Verification items for the finished model (mm, model axes). Face numbers are marked on the shaded views. A direction names the side the tool comes from. Round coordinates to 2 decimals unless told otherwise and drop trailing zeros. Write each loop counter-clockwise with the first axis right and the second up, starting at its lowest first coordinate (ties: lowest second). Pieces come first, ordered by that corner, then holes. Notation, with made-up numbers: (20, -19) - (54, -19) arc R4 ccw to (54, -12) - close; hole circle Ø3 at (-4, 39). An arc over 180 degrees is marked (long way). Answer as a JSON object with one key per item and string values.
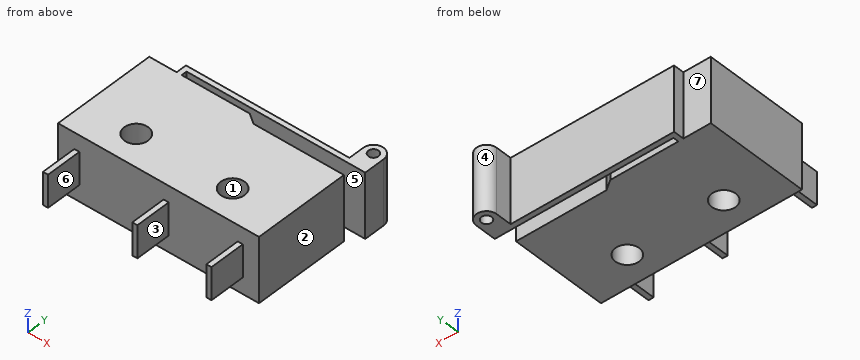
```python
from build123d import *

# Parameters (mm, degrees)
SKETCH1_R           = 1.175
SKETCH1_R_2         = 0.5
BOSS_EXTRUDE1_DEPTH = 6.4
SKETCH2_W           = 1.6
SKETCH2_H           = 3.5
CUT_EXTRUDE1_DEPTH  = 21.8
CUT_EXTRUDE2_DEPTH  = 7.4


with BuildPart() as part:
    # Sketch1 → Boss-Extrude1 (new body)
    with BuildSketch(Plane.XY):
        with BuildLine():
            Line((2.1, 0), (10.4, 0))
            Line((10.4, 0), (10.4, -3.5))
            Line((10.4, -3.5), (10.9, -3.5))
            Line((10.9, -3.5), (10.9, 0))
            Line((10.9, 0), (17.7, 0))
            Line((17.7, 0), (17.7, -3.5))
            Line((17.7, -3.5), (18.2, -3.5))
            Line((18.2, -3.5), (18.2, 0))
            Line((18.2, 0), (19.8, 0))
            Line((19.8, 0), (19.8, 10.2))
            Line((19.8, 10.2), (3.195717589, 10.2))
            Line((3.195717589, 10.2), (3.195717589, 10.746282688))
            Line((3.195717589, 10.746282688), (20.8, 10.746282688))
            Line((20.8, 10.746282688), (20.8, 12.80322859))
            ThreePointArc((20.8, 12.80322859), (19.8, 13.80322859), (18.8, 12.80322859))
            Line((18.8, 12.80322859), (18.8, 11.246282688))
            Line((18.8, 11.246282688), (2.695717589, 11.246282688))
            Line((2.695717589, 11.246282688), (2.695717589, 10.2))
            Line((2.695717589, 10.2), (0, 10.2))
            Line((0, 10.2), (0, 0))
            Line((0, 0), (1.6, 0))
            Line((1.6, 0), (1.6, -3.5))
            Line((1.6, -3.5), (2.1, -3.5))
            Line((2.1, -3.5), (2.1, 0))
        make_face()
        with Locations((5.15, 2.9)):
            Circle(SKETCH1_R, mode=Mode.SUBTRACT)
        with Locations((14.65, 2.9)):
            Circle(SKETCH1_R, mode=Mode.SUBTRACT)
        with Locations((19.8, 12.80322859)):
            Circle(SKETCH1_R_2, mode=Mode.SUBTRACT)
    extrude(amount=BOSS_EXTRUDE1_DEPTH)

    # Sketch2 → Cut-Extrude1 (cut, through all)
    with BuildSketch(Plane.ZY):
        with Locations((0.8, -1.75)):
            Rectangle(SKETCH2_W, SKETCH2_H)
        with Locations((5.6, -1.75)):
            Rectangle(SKETCH2_W, SKETCH2_H)
    extrude(amount=-CUT_EXTRUDE1_DEPTH, mode=Mode.SUBTRACT)

    # Sketch3 → Cut-Extrude2 (cut, through all)
    with BuildSketch(Plane.XY.offset(6.4)):
        Polygon((19.8, 9.5), (10.9, 9.5), (9.9, 10.2), (19.8, 10.2), align=None)
    extrude(amount=-CUT_EXTRUDE2_DEPTH, mode=Mode.SUBTRACT)


solid = part.part
```
1. Go/stop test with flat-tipped pins: pin 1 (2.5 mm diameter, centred on y = -2, z = 2.5, fed in from +X); pin 2 (3.5 mm diameter, centred on y = -1, z = 3, fed in from +X); pin 3 (3.5 mm diameter, centred on y = -1.5, z = 3.5, fed in from -X); pin 4 (1 mm diameter, centred on x = 18, z = 1, fed in from +Y). Record where each tip stops, or that it passes through.
Completed:
{"pin 1": "stops at x = 18.2", "pin 2": "stops at x = 19.8", "pin 3": "stops at x = 0", "pin 4": "stops at y = 11.25"}
2. Cross-section at D-D (y = 2.9). Record the boundary of the cut face in (x, z) (3 decimals).
Completed:
{"outline": "(0, 0) - (3.975, 0) - (3.975, 6.4) - (0, 6.4) - close; (6.325, 0) - (13.475, 0) - (13.475, 6.4) - (6.325, 6.4) - close; (15.825, 0) - (19.8, 0) - (19.8, 6.4) - (15.825, 6.4) - close"}
3. Cross-section at C-C (x = 13). Record the boundary of the cut face in (y, z), plus the area to 3 significant figures.
Completed:
{"outline": "(0, 0) - (9.5, 0) - (9.5, 6.4) - (0, 6.4) - close; (10.75, 0) - (11.25, 0) - (11.25, 6.4) - (10.75, 6.4) - close", "area": "64.0 mm^2"}
4. Mould release check, pull along X, two halves, no side actions. Record for the marked faces 1, 2, 3 and 4: released by +X, released by -X, zero draft, split by the parting line, or undercut.
Completed:
{"face 1": "undercut", "face 2": "released by +X", "face 3": "undercut", "face 4": "split by the parting line"}
5. Cross-section at A-A (x = 5.15). Record the boundary of the cut face in (y, z) (3 decimals), plus the area to 3 significant figures.
Completed:
{"outline": "(0, 0) - (1.725, 0) - (1.725, 6.4) - (0, 6.4) - close; (4.075, 0) - (10.2, 0) - (10.2, 6.4) - (4.075, 6.4) - close; (10.746, 0) - (11.246, 0) - (11.246, 6.4) - (10.746, 6.4) - close", "area": "53.4 mm^2"}
6. Material ranges on probe 1 along X at (y, z) = (3, 1); probe 2 along Y at (x, z) = (14.65, 4.25) (3 decimals); probe 3 along X at (y, z) = (-2, 3.5), recorded low to high. Write a range as from..to.
Completed:
{"probe 1": "x = 0..3.98, 6.32..13.48, 15.82..19.8", "probe 2": "y = 0..1.725, 4.075..9.5, 10.746..11.246", "probe 3": "x = 1.6..2.1, 10.4..10.9, 17.7..18.2"}
7. Access from +Z, -Z, +X, -X, +Y, -Y to the whole of each face (thin tool, end or side, straight path). Record for the marked faces 5, 6 and 7.
Completed:
{"face 5": "+Z, -Z, +X", "face 6": "+Z, -Z, -Y", "face 7": "+Z, -Z, -X, +Y"}
8. Cross-section at B-B (z = 3). Count the separate pieces of the cut face and the enclosed holes in it, plus the area to 3 significant figures.
Completed:
{"separate pieces": "1", "enclosed holes": "3", "area": "205 mm^2"}
